Geometry check sheet. Reference: the model listing, model coordinates, mm. Round coordinates to 2 decimals unless told otherwise and drop trailing zeros. Order: outer loops, then holes, each group sorted by start corner. A loop starts at its lowest first (then second) coordinate and runs counter-clockwise, first axis right, second up. Notation, with made-up numbers: (87, 34) -> (118, 34) arc R20 cw to (118, 64) -> close; hole circle Ø9 at (-28, 42). An arc over 180 degrees is marked (long way). Use a Markdown table: item, result. Add a question column.
Item 1: Sectioned sample at C-C, the plane y = 3.75. State how many separate pieces and enclosed holes the cut face has, and give its area (3 significant figures).
Item 2: Material ranges on probe 1 along Z at (x, y) = (-75.85, 4.5); probe 2 along Z at (x, y) = (-309, 7); probe 3 along X at (y, z) = (7, 20), recorded low to high. Write a range as [from, to].
Item 3: Sectioned sample at A-A, the plane x = 101.5. Record the cut outline in (y, z), and give its area (4 significant figures).
Item 4: Gauge pin test, flat end, axial feed: pin 1 Ø2 at (x, z) = (493.4, -45.75) entering from -Y. Record the tip position at first contact, or that the pin passes through.
Item 5: Sectioned sample at B-B, the plane z = 29. Record the cut outline in (x, y).
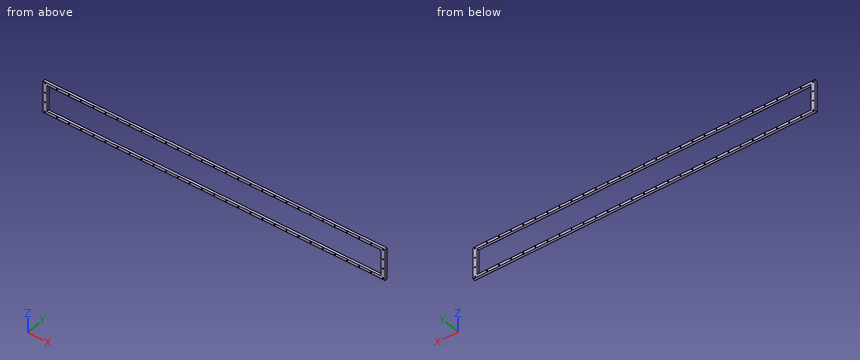
from build123d import *

# Parameters (mm, degrees)
SKETCH2_W                = 1075
SKETCH2_H                = 100
SKETCH2_W_2              = 1050
SKETCH2_H_2              = 83
BOSS_EXTRUDE1_DEPTH      = 7.5
CUT_EXTRUDE1_START       = -8.5
SKETCH3_R                = 1.7
CUT_EXTRUDE1_DEPTH       = 9.5
LPATTERN1_COUNT          = 4
LPATTERN1_PITCH          = 30.425
LPATTERN2_COUNT          = 29
LPATTERN2_PITCH          = 37.95
MIRROR1_START            = -8.5
MIRROR1_COPY_1_SKETCH_R  = 1.7
MIRROR1_COPY_1_DEPTH     = 9.5
MIRROR1_COPY_2_SKETCH_R  = 1.7
MIRROR1_COPY_2_DEPTH     = 9.5
MIRROR1_COPY_3_SKETCH_R  = 1.7
MIRROR1_COPY_3_DEPTH     = 9.5
MIRROR1_COPY_4_SKETCH_R  = 1.7
MIRROR1_COPY_4_DEPTH     = 9.5
MIRROR1_COPY_5_SKETCH_R  = 1.7
MIRROR1_COPY_5_DEPTH     = 9.5
MIRROR1_COPY_6_SKETCH_R  = 1.7
MIRROR1_COPY_6_DEPTH     = 9.5
MIRROR1_COPY_7_SKETCH_R  = 1.7
MIRROR1_COPY_7_DEPTH     = 9.5
MIRROR1_COPY_8_SKETCH_R  = 1.7
MIRROR1_COPY_8_DEPTH     = 9.5
MIRROR1_COPY_9_SKETCH_R  = 1.7
MIRROR1_COPY_9_DEPTH     = 9.5
MIRROR1_COPY_10_SKETCH_R = 1.7
MIRROR1_COPY_10_DEPTH    = 9.5
MIRROR1_COPY_11_SKETCH_R = 1.7
MIRROR1_COPY_11_DEPTH    = 9.5
MIRROR1_COPY_12_SKETCH_R = 1.7
MIRROR1_COPY_12_DEPTH    = 9.5
MIRROR1_COPY_13_SKETCH_R = 1.7
MIRROR1_COPY_13_DEPTH    = 9.5
MIRROR1_COPY_14_SKETCH_R = 1.7
MIRROR1_COPY_14_DEPTH    = 9.5
MIRROR1_COPY_15_SKETCH_R = 1.7
MIRROR1_COPY_15_DEPTH    = 9.5
MIRROR1_COPY_16_SKETCH_R = 1.7
MIRROR1_COPY_16_DEPTH    = 9.5
MIRROR1_COPY_17_SKETCH_R = 1.7
MIRROR1_COPY_17_DEPTH    = 9.5
MIRROR1_COPY_18_SKETCH_R = 1.7
MIRROR1_COPY_18_DEPTH    = 9.5
MIRROR1_COPY_19_SKETCH_R = 1.7
MIRROR1_COPY_19_DEPTH    = 9.5
MIRROR1_COPY_20_SKETCH_R = 1.7
MIRROR1_COPY_20_DEPTH    = 9.5
MIRROR1_COPY_21_SKETCH_R = 1.7
MIRROR1_COPY_21_DEPTH    = 9.5
MIRROR1_COPY_22_SKETCH_R = 1.7
MIRROR1_COPY_22_DEPTH    = 9.5
MIRROR1_COPY_23_SKETCH_R = 1.7
MIRROR1_COPY_23_DEPTH    = 9.5
MIRROR1_COPY_24_SKETCH_R = 1.7
MIRROR1_COPY_24_DEPTH    = 9.5
MIRROR1_COPY_25_SKETCH_R = 1.7
MIRROR1_COPY_25_DEPTH    = 9.5
MIRROR1_COPY_26_SKETCH_R = 1.7
MIRROR1_COPY_26_DEPTH    = 9.5
MIRROR1_COPY_27_SKETCH_R = 1.7
MIRROR1_COPY_27_DEPTH    = 9.5
MIRROR1_COPY_28_SKETCH_R = 1.7
MIRROR1_COPY_28_DEPTH    = 9.5
MIRROR2_START            = -8.5
MIRROR2_COPY_1_SKETCH_R  = 1.7
MIRROR2_COPY_1_DEPTH     = 9.5
MIRROR2_COPY_2_SKETCH_R  = 1.7
MIRROR2_COPY_2_DEPTH     = 9.5
MIRROR2_COPY_3_SKETCH_R  = 1.7
MIRROR2_COPY_3_DEPTH     = 9.5


with BuildPart() as part:
    # Sketch2 → Boss-Extrude1 (new body)
    with BuildSketch(Plane(origin=(0, 0, 0), x_dir=(1, 0, 0), z_dir=(0, 1, 0))):
        Rectangle(SKETCH2_W, SKETCH2_H)
        Rectangle(SKETCH2_W_2, SKETCH2_H_2, mode=Mode.SUBTRACT)
    extrude(amount=BOSS_EXTRUDE1_DEPTH)

    # Sketch3 → Cut-Extrude1 (cut)
    with BuildSketch(Plane.XZ.offset(CUT_EXTRUDE1_START)):
        with Locations((-531.25, 45.75)):
            Circle(SKETCH3_R)
    cut_extrude1 = extrude(amount=CUT_EXTRUDE1_DEPTH, mode=Mode.SUBTRACT)

    # LPattern1: Cut-Extrude1 ×4
    with Locations(*[(0, 0, -i * LPATTERN1_PITCH) for i in range(1, LPATTERN1_COUNT)]):
        add(cut_extrude1, mode=Mode.SUBTRACT)

    # LPattern2: Cut-Extrude1 ×29
    with Locations(*[(i * LPATTERN2_PITCH, 0, 0) for i in range(1, LPATTERN2_COUNT)]):
        add(cut_extrude1, mode=Mode.SUBTRACT)

    # Mirror1: Cut-Extrude1 across plane
    add(cut_extrude1.mirror(Plane.XY), mode=Mode.SUBTRACT)

    # Mirror1 copy 1 sketch → Mirror1 copy 1 (cut)
    with BuildSketch(Plane(origin=(37.95, 0, 0), x_dir=(1, 0, 0), z_dir=(0, -1, 0)).offset(MIRROR1_START)):
        with Locations((-531.25, -45.75)):
            Circle(MIRROR1_COPY_1_SKETCH_R)
    extrude(amount=MIRROR1_COPY_1_DEPTH, mode=Mode.SUBTRACT)

    # Mirror1 copy 2 sketch → Mirror1 copy 2 (cut)
    with BuildSketch(Plane(origin=(75.9, 0, 0), x_dir=(1, 0, 0), z_dir=(0, -1, 0)).offset(MIRROR1_START)):
        with Locations((-531.25, -45.75)):
            Circle(MIRROR1_COPY_2_SKETCH_R)
    extrude(amount=MIRROR1_COPY_2_DEPTH, mode=Mode.SUBTRACT)

    # Mirror1 copy 3 sketch → Mirror1 copy 3 (cut)
    with BuildSketch(Plane(origin=(113.85, 0, 0), x_dir=(1, 0, 0), z_dir=(0, -1, 0)).offset(MIRROR1_START)):
        with Locations((-531.25, -45.75)):
            Circle(MIRROR1_COPY_3_SKETCH_R)
    extrude(amount=MIRROR1_COPY_3_DEPTH, mode=Mode.SUBTRACT)

    # Mirror1 copy 4 sketch → Mirror1 copy 4 (cut)
    with BuildSketch(Plane(origin=(151.8, 0, 0), x_dir=(1, 0, 0), z_dir=(0, -1, 0)).offset(MIRROR1_START)):
        with Locations((-531.25, -45.75)):
            Circle(MIRROR1_COPY_4_SKETCH_R)
    extrude(amount=MIRROR1_COPY_4_DEPTH, mode=Mode.SUBTRACT)

    # Mirror1 copy 5 sketch → Mirror1 copy 5 (cut)
    with BuildSketch(Plane(origin=(189.75, 0, 0), x_dir=(1, 0, 0), z_dir=(0, -1, 0)).offset(MIRROR1_START)):
        with Locations((-531.25, -45.75)):
            Circle(MIRROR1_COPY_5_SKETCH_R)
    extrude(amount=MIRROR1_COPY_5_DEPTH, mode=Mode.SUBTRACT)

    # Mirror1 copy 6 sketch → Mirror1 copy 6 (cut)
    with BuildSketch(Plane(origin=(227.7, 0, 0), x_dir=(1, 0, 0), z_dir=(0, -1, 0)).offset(MIRROR1_START)):
        with Locations((-531.25, -45.75)):
            Circle(MIRROR1_COPY_6_SKETCH_R)
    extrude(amount=MIRROR1_COPY_6_DEPTH, mode=Mode.SUBTRACT)

    # Mirror1 copy 7 sketch → Mirror1 copy 7 (cut)
    with BuildSketch(Plane(origin=(265.65, 0, 0), x_dir=(1, 0, 0), z_dir=(0, -1, 0)).offset(MIRROR1_START)):
        with Locations((-531.25, -45.75)):
            Circle(MIRROR1_COPY_7_SKETCH_R)
    extrude(amount=MIRROR1_COPY_7_DEPTH, mode=Mode.SUBTRACT)

    # Mirror1 copy 8 sketch → Mirror1 copy 8 (cut)
    with BuildSketch(Plane(origin=(303.6, 0, 0), x_dir=(1, 0, 0), z_dir=(0, -1, 0)).offset(MIRROR1_START)):
        with Locations((-531.25, -45.75)):
            Circle(MIRROR1_COPY_8_SKETCH_R)
    extrude(amount=MIRROR1_COPY_8_DEPTH, mode=Mode.SUBTRACT)

    # Mirror1 copy 9 sketch → Mirror1 copy 9 (cut)
    with BuildSketch(Plane(origin=(341.55, 0, 0), x_dir=(1, 0, 0), z_dir=(0, -1, 0)).offset(MIRROR1_START)):
        with Locations((-531.25, -45.75)):
            Circle(MIRROR1_COPY_9_SKETCH_R)
    extrude(amount=MIRROR1_COPY_9_DEPTH, mode=Mode.SUBTRACT)

    # Mirror1 copy 10 sketch → Mirror1 copy 10 (cut)
    with BuildSketch(Plane(origin=(379.5, 0, 0), x_dir=(1, 0, 0), z_dir=(0, -1, 0)).offset(MIRROR1_START)):
        with Locations((-531.25, -45.75)):
            Circle(MIRROR1_COPY_10_SKETCH_R)
    extrude(amount=MIRROR1_COPY_10_DEPTH, mode=Mode.SUBTRACT)

    # Mirror1 copy 11 sketch → Mirror1 copy 11 (cut)
    with BuildSketch(Plane(origin=(417.45, 0, 0), x_dir=(1, 0, 0), z_dir=(0, -1, 0)).offset(MIRROR1_START)):
        with Locations((-531.25, -45.75)):
            Circle(MIRROR1_COPY_11_SKETCH_R)
    extrude(amount=MIRROR1_COPY_11_DEPTH, mode=Mode.SUBTRACT)

    # Mirror1 copy 12 sketch → Mirror1 copy 12 (cut)
    with BuildSketch(Plane(origin=(455.4, 0, 0), x_dir=(1, 0, 0), z_dir=(0, -1, 0)).offset(MIRROR1_START)):
        with Locations((-531.25, -45.75)):
            Circle(MIRROR1_COPY_12_SKETCH_R)
    extrude(amount=MIRROR1_COPY_12_DEPTH, mode=Mode.SUBTRACT)

    # Mirror1 copy 13 sketch → Mirror1 copy 13 (cut)
    with BuildSketch(Plane(origin=(493.35, 0, 0), x_dir=(1, 0, 0), z_dir=(0, -1, 0)).offset(MIRROR1_START)):
        with Locations((-531.25, -45.75)):
            Circle(MIRROR1_COPY_13_SKETCH_R)
    extrude(amount=MIRROR1_COPY_13_DEPTH, mode=Mode.SUBTRACT)

    # Mirror1 copy 14 sketch → Mirror1 copy 14 (cut)
    with BuildSketch(Plane(origin=(531.3, 0, 0), x_dir=(1, 0, 0), z_dir=(0, -1, 0)).offset(MIRROR1_START)):
        with Locations((-531.25, -45.75)):
            Circle(MIRROR1_COPY_14_SKETCH_R)
    extrude(amount=MIRROR1_COPY_14_DEPTH, mode=Mode.SUBTRACT)

    # Mirror1 copy 15 sketch → Mirror1 copy 15 (cut)
    with BuildSketch(Plane(origin=(569.25, 0, 0), x_dir=(1, 0, 0), z_dir=(0, -1, 0)).offset(MIRROR1_START)):
        with Locations((-531.25, -45.75)):
            Circle(MIRROR1_COPY_15_SKETCH_R)
    extrude(amount=MIRROR1_COPY_15_DEPTH, mode=Mode.SUBTRACT)

    # Mirror1 copy 16 sketch → Mirror1 copy 16 (cut)
    with BuildSketch(Plane(origin=(607.2, 0, 0), x_dir=(1, 0, 0), z_dir=(0, -1, 0)).offset(MIRROR1_START)):
        with Locations((-531.25, -45.75)):
            Circle(MIRROR1_COPY_16_SKETCH_R)
    extrude(amount=MIRROR1_COPY_16_DEPTH, mode=Mode.SUBTRACT)

    # Mirror1 copy 17 sketch → Mirror1 copy 17 (cut)
    with BuildSketch(Plane(origin=(645.15, 0, 0), x_dir=(1, 0, 0), z_dir=(0, -1, 0)).offset(MIRROR1_START)):
        with Locations((-531.25, -45.75)):
            Circle(MIRROR1_COPY_17_SKETCH_R)
    extrude(amount=MIRROR1_COPY_17_DEPTH, mode=Mode.SUBTRACT)

    # Mirror1 copy 18 sketch → Mirror1 copy 18 (cut)
    with BuildSketch(Plane(origin=(683.1, 0, 0), x_dir=(1, 0, 0), z_dir=(0, -1, 0)).offset(MIRROR1_START)):
        with Locations((-531.25, -45.75)):
            Circle(MIRROR1_COPY_18_SKETCH_R)
    extrude(amount=MIRROR1_COPY_18_DEPTH, mode=Mode.SUBTRACT)

    # Mirror1 copy 19 sketch → Mirror1 copy 19 (cut)
    with BuildSketch(Plane(origin=(721.05, 0, 0), x_dir=(1, 0, 0), z_dir=(0, -1, 0)).offset(MIRROR1_START)):
        with Locations((-531.25, -45.75)):
            Circle(MIRROR1_COPY_19_SKETCH_R)
    extrude(amount=MIRROR1_COPY_19_DEPTH, mode=Mode.SUBTRACT)

    # Mirror1 copy 20 sketch → Mirror1 copy 20 (cut)
    with BuildSketch(Plane(origin=(759, 0, 0), x_dir=(1, 0, 0), z_dir=(0, -1, 0)).offset(MIRROR1_START)):
        with Locations((-531.25, -45.75)):
            Circle(MIRROR1_COPY_20_SKETCH_R)
    extrude(amount=MIRROR1_COPY_20_DEPTH, mode=Mode.SUBTRACT)

    # Mirror1 copy 21 sketch → Mirror1 copy 21 (cut)
    with BuildSketch(Plane(origin=(796.95, 0, 0), x_dir=(1, 0, 0), z_dir=(0, -1, 0)).offset(MIRROR1_START)):
        with Locations((-531.25, -45.75)):
            Circle(MIRROR1_COPY_21_SKETCH_R)
    extrude(amount=MIRROR1_COPY_21_DEPTH, mode=Mode.SUBTRACT)

    # Mirror1 copy 22 sketch → Mirror1 copy 22 (cut)
    with BuildSketch(Plane(origin=(834.9, 0, 0), x_dir=(1, 0, 0), z_dir=(0, -1, 0)).offset(MIRROR1_START)):
        with Locations((-531.25, -45.75)):
            Circle(MIRROR1_COPY_22_SKETCH_R)
    extrude(amount=MIRROR1_COPY_22_DEPTH, mode=Mode.SUBTRACT)

    # Mirror1 copy 23 sketch → Mirror1 copy 23 (cut)
    with BuildSketch(Plane(origin=(872.85, 0, 0), x_dir=(1, 0, 0), z_dir=(0, -1, 0)).offset(MIRROR1_START)):
        with Locations((-531.25, -45.75)):
            Circle(MIRROR1_COPY_23_SKETCH_R)
    extrude(amount=MIRROR1_COPY_23_DEPTH, mode=Mode.SUBTRACT)

    # Mirror1 copy 24 sketch → Mirror1 copy 24 (cut)
    with BuildSketch(Plane(origin=(910.8, 0, 0), x_dir=(1, 0, 0), z_dir=(0, -1, 0)).offset(MIRROR1_START)):
        with Locations((-531.25, -45.75)):
            Circle(MIRROR1_COPY_24_SKETCH_R)
    extrude(amount=MIRROR1_COPY_24_DEPTH, mode=Mode.SUBTRACT)

    # Mirror1 copy 25 sketch → Mirror1 copy 25 (cut)
    with BuildSketch(Plane(origin=(948.75, 0, 0), x_dir=(1, 0, 0), z_dir=(0, -1, 0)).offset(MIRROR1_START)):
        with Locations((-531.25, -45.75)):
            Circle(MIRROR1_COPY_25_SKETCH_R)
    extrude(amount=MIRROR1_COPY_25_DEPTH, mode=Mode.SUBTRACT)

    # Mirror1 copy 26 sketch → Mirror1 copy 26 (cut)
    with BuildSketch(Plane(origin=(986.7, 0, 0), x_dir=(1, 0, 0), z_dir=(0, -1, 0)).offset(MIRROR1_START)):
        with Locations((-531.25, -45.75)):
            Circle(MIRROR1_COPY_26_SKETCH_R)
    extrude(amount=MIRROR1_COPY_26_DEPTH, mode=Mode.SUBTRACT)

    # Mirror1 copy 27 sketch → Mirror1 copy 27 (cut)
    with BuildSketch(Plane(origin=(1024.65, 0, 0), x_dir=(1, 0, 0), z_dir=(0, -1, 0)).offset(MIRROR1_START)):
        with Locations((-531.25, -45.75)):
            Circle(MIRROR1_COPY_27_SKETCH_R)
    extrude(amount=MIRROR1_COPY_27_DEPTH, mode=Mode.SUBTRACT)

    # Mirror1 copy 28 sketch → Mirror1 copy 28 (cut)
    with BuildSketch(Plane(origin=(1062.6, 0, 0), x_dir=(1, 0, 0), z_dir=(0, -1, 0)).offset(MIRROR1_START)):
        with Locations((-531.25, -45.75)):
            Circle(MIRROR1_COPY_28_SKETCH_R)
    extrude(amount=MIRROR1_COPY_28_DEPTH, mode=Mode.SUBTRACT)

    # Mirror2: Cut-Extrude1 across plane
    add(cut_extrude1.mirror(Plane(origin=(0, 0, 0), x_dir=(0, 0, 1), z_dir=(1, 0, 0))), mode=Mode.SUBTRACT)

    # Mirror2 copy 1 sketch → Mirror2 copy 1 (cut)
    with BuildSketch(Plane(origin=(0, 0, -30.425), x_dir=(-1, 0, 0), z_dir=(0, -1, 0)).offset(MIRROR2_START)):
        with Locations((-531.25, -45.75)):
            Circle(MIRROR2_COPY_1_SKETCH_R)
    extrude(amount=MIRROR2_COPY_1_DEPTH, mode=Mode.SUBTRACT)

    # Mirror2 copy 2 sketch → Mirror2 copy 2 (cut)
    with BuildSketch(Plane(origin=(0, 0, -60.85), x_dir=(-1, 0, 0), z_dir=(0, -1, 0)).offset(MIRROR2_START)):
        with Locations((-531.25, -45.75)):
            Circle(MIRROR2_COPY_2_SKETCH_R)
    extrude(amount=MIRROR2_COPY_2_DEPTH, mode=Mode.SUBTRACT)

    # Mirror2 copy 3 sketch → Mirror2 copy 3 (cut)
    with BuildSketch(Plane(origin=(0, 0, -91.275), x_dir=(-1, 0, 0), z_dir=(0, -1, 0)).offset(MIRROR2_START)):
        with Locations((-531.25, -45.75)):
            Circle(MIRROR2_COPY_3_SKETCH_R)
    extrude(amount=MIRROR2_COPY_3_DEPTH, mode=Mode.SUBTRACT)


solid = part.part
Found:
| question | item | result |
|---|---|---|
| 1 | separate pieces | 1 |
| 1 | enclosed holes | 63 |
| 1 | area | 19,800 mm2 |
| 2 | probe 1 | z = [-50, -47.45], [-44.05, -41.5], [41.5, 44.05], [47.45, 50] |
| 2 | probe 2 | z = [-50, -41.5], [41.5, 50] |
| 2 | probe 3 | x = [-537.5, -525], [525, 537.5] |
| 3 | outline | (0, -50) -> (7.5, -50) -> (7.5, -41.5) -> (0, -41.5) -> close; (0, 41.5) -> (7.5, 41.5) -> (7.5, 50) -> (0, 50) -> close |
| 3 | area | 127.5 mm2 |
| 4 | pin 1 | passes through |
| 5 | outline | (-537.5, 0) -> (-525, 0) -> (-525, 7.5) -> (-537.5, 7.5) -> close; (525, 0) -> (537.5, 0) -> (537.5, 7.5) -> (525, 7.5) -> close |
